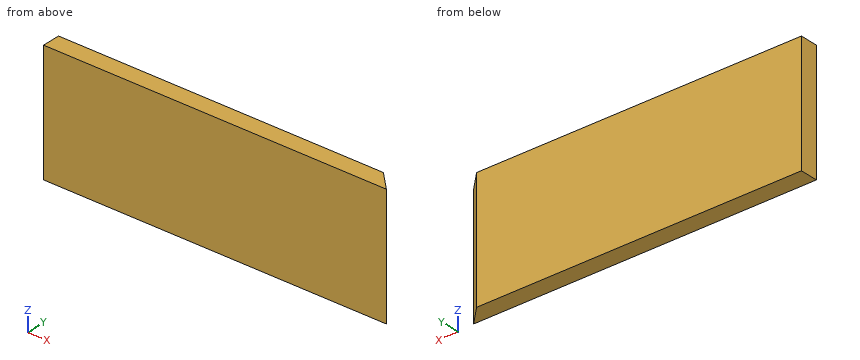
```python
from build123d import *

# Parameters (mm, degrees)
F0_W     = 361.95
F0_H     = 127
F1_DEPTH = 19.05
F2_SIZE2 = 19.04999
F2_SIZE  = 19.04999


# Not quite as in the source:
# - a fillet or chamfer is up to 0.001 mm smaller than in the source, because OpenCascade refuses the exact size


with BuildPart() as f1:
    # F0 (on Front) → F1 (new body)
    with BuildSketch(Plane.XZ):
        with Locations((29.6110501051, 33.5559173692)):
            Rectangle(F0_W, F0_H)
    extrude(amount=F1_DEPTH)

    # F2 (size 19.05 and 19.05 in the source; OpenCascade refuses exactly that, so slightly less here)
    f2_edges = [f1.edges().sort_by_distance(p)[0] for p in [
        (210.58605, 0, 33.555917),
    ]]
    chamfer(f2_edges, length=F2_SIZE, length2=F2_SIZE2)


solid = f1.part
```
Check sheet for the modelled part. Datum: model origin and axes. Units: mm. Round coordinates to 2 decimals unless told otherwise and drop trailing zeros. Order: outer loops, then holes, each group sorted by start corner. A loop starts at its lowest first (then second) coordinate and runs counter-clockwise, first axis right, second up.
1) Section check B-B (y = -3). Record the boundary of the cut face in (x, z), and give its area (3 significant figures).
2) Go/stop test with flat-tipped pins: pin 1 Ø5 at (y, z) = (-10.5, 14) entering from +X; pin 2 Ø5 at (y, z) = (-13.5, 58.5) entering from +X. Record where each tip stops, or that it passes through.
3) Scan lines: line 1 (X direction, y = -8.75, z = 39); line 2 (X direction, y = -17.75, z = 82). Record each from-to range of solid material in increasing order.
Result:
1. outline: (-151.36, -29.94) - (194.54, -29.94) - (194.54, 97.06) - (-151.36, 97.06) - close
1. area: 43,900 mm2
2. pin 1: stops at x = 204.54
2. pin 2: stops at x = 207.54
3. line 1: x = -151.36 to 200.29
3. line 2: x = -151.36 to 209.29
